Geometry: final body of the model. Coordinates: model frame, mm. A direction names the side the tool comes from. Give positions to 0.01 mm unless a question says otherwise; leave off trailing zeros. Order: outer loops, then holes, each group sorted by start corner. A loop starts at its lowest first (then second) coordinate and runs counter-clockwise, first axis right, second up. Notation, with made-up numbers: (-4, -23) -> (40, -23) arc R17 ccw to (40, 3) -> close; hole circle Ø11 at (-23, 74.25). An arc over 180 degrees is marked (long way). One line per question, with ' | ' between items.
Autodesk Inventor part; units mm, degrees
ref_plane "Work Plane2" through (0, 0, -18.4174) normal (0, 0, 1) x (1, 0, 0)
ref_plane "YZ Plane" through (0, 0, 0) normal (1, 0, 0) x (0, 1, 0)
ref_plane "XZ Plane" through (0, 0, 0) normal (0, 1, 0) x (-1, 0, 0)
sketch "Sketch1" plane through (0, 0, 0) normal (0, 1, 0) x (-1, 0, 0)
  line L0 (60.406, 25.6071) -> (-60.406, 25.6071)
  line L1 (-60.406, 25.6071) -> (-60.406, -25.6071)
  line L2 (-60.406, -25.6071) -> (60.406, -25.6071)
  line L3 (60.406, -25.6071) -> (60.406, 25.6071)
  line L4 (60.406, 25.6071) -> (-60.406, -25.6071) construction
  line L5 (-60.406, 25.6071) -> (60.406, -25.6071) construction
  line L6 (-57.406, 25.6071) -> (-57.406, -25.6071)
  line L7 (57.406, -25.6071) -> (57.406, 25.6071)
  line L8 (57.406, 23.5058) -> (55.4493, 23.5058)
  line L9 (-55.4493, 23.5058) -> (-57.406, 23.5058)
  line L10 (-57.406, -33.4947) -> (-79.0126, -33.4947)
  line L11 (79.0126, -33.4947) -> (57.406, -33.4947)
  point P0 (0, 0)
  dimension "d0" = 120.812
  dimension "d1" = 51.2141
  dimension "d8" = 3
  dimension "d9" = 3
  dimension "d10" = 114.812
extrude "Extrusion1" add sketch "Sketch1" along normal blind 3
extrude "Extrusion2" add sketch "Sketch1" along normal blind 63 contours L3 L2 L7 L0 | L6 L2 L1 L0
ref_plane "Work Plane2" through (0, 0, -18.4174) normal (0, 0, 1) x (1, 0, 0)
sketch "Sketch2" plane through (0, 0, 0) normal (0, -1, 0) x (1, 0, 0)
  circle A0 centre (-50.5968, 0.5202) radius 1.75
  circle A1 centre (-28.0003, -13.4843) radius 1.75
  circle A2 centre (50.5962, 0.5202) radius 1.75
  circle A3 centre (27.9997, -13.4843) radius 1.75
  circle A4 centre (27.9997, -13.4843) radius 1.75
  circle A5 centre (50.5962, 0.5202) radius 1.75
  circle A6 centre (-28.0003, -13.4843) radius 1.75
  circle A7 centre (-50.5968, 0.5202) radius 1.75
  point P0 (0, 0)
  dimension "d12" = 3.5
  dimension "d13" = 3.5
  dimension "d14" = 3.5
  dimension "d15" = 3.5
extrude "Extrusion3" cut sketch "Sketch2" against normal up to next
sketch "Sketch4" plane through (0, 63, 0) normal (0, 1, 0) x (1, 0, 0)
  line L0 (-60.406, -8.75) -> (-56.906, -8.75)
  line L1 (-56.906, -8.75) -> (-56.906, 8.75)
  line L2 (-56.906, 8.75) -> (-60.406, 8.75)
  line L3 (-60.406, -8.75) -> (-60.406, 8.75)
  line L4 (0, 0) -> (0, 8.75)
  line L5 (60.406, -8.75) -> (56.906, -8.75)
  line L6 (56.906, -8.75) -> (56.906, 8.75)
  line L7 (56.906, 8.75) -> (60.406, 8.75)
  line L8 (60.406, -8.75) -> (60.406, 8.75)
  point P0 (-60.406, 0)
  point P1 (60.406, 0)
  dimension "d18" = 17.5
extrude "Extrusion4" cut sketch "Sketch4" against normal blind 3
sketch "Sketch6" plane through (0, 0, 0) normal (0, -1, 0) x (1, 0, 0)
  circle A0 centre (-32.4423, 8.2996) radius 1.5
  circle A1 centre (32.4417, 8.2996) radius 1.5
  point P0 (0, 0)
extrude "Extrusion5" cut sketch "Sketch6" against normal up to next
sketch "Sketch9" plane through (60.406, 0, 25.6071) normal (1, 0, 0) x (0, 0, -1)
  circle A0 centre (3, 59.0338) radius 1
  circle A1 centre (3, 38.0338) radius 1
  circle A2 centre (48.2141, 59.0338) radius 1
  circle A3 centre (48.2141, 38.0338) radius 1
  point P0 (25.6071, 0)
extrude "Extrusion7" cut sketch "Sketch9" against normal blind 200
sketch "Sketch10" plane through (0, 0, 0) normal (0, -1, 0) x (1, 0, 0)
  circle A0 centre (-28.0003, -13.4843) radius 1.75
  circle A1 centre (27.9997, -13.4843) radius 1.75
  line L0 (53.5962, 73.5112) -> (-53.5968, 73.5112)
  line L1 (-24.5003, -13.4843) -> (24.4997, -13.4843)
  line L2 (24.4997, 73.5112) -> (-24.5003, 73.5112)
  line L3 (-24.5003, -13.4843) -> (-24.5003, -2.4798)
  line L4 (-24.5003, -13.4843) -> (-13.4958, -13.4843) construction
  line L5 (-24.5003, -2.4798) -> (24.4997, -2.4798)
  line L6 (24.4997, -13.4843) -> (24.4997, -2.4798)
  point P0 (0, 0)
  dimension "d39" = 90
extrude "Extrusion8" cut sketch "Sketch10" against normal up to next contours L3 L5 L6 L1
sketch "Sketch11" plane through (0, 0, 0) normal (0, -1, 0) x (1, 0, 0)
  circle A0 centre (-38.0003, 13.0422) radius 1.75
  circle A1 centre (-14.0003, 13.0422) radius 1.75
  line L0 (-36.0003, -4.4688) -> (-36.0003, 50.5312)
  line L1 (-16.0003, 50.5312) -> (-16.0003, -4.4688)
  line L2 (-34.6078, 15.0422) -> (34.6072, 15.0422)
  point P0 (0, 0)
  dimension "d31" = 3.5
  dimension "d32" = 3.5
  dimension "d33" = 2
  dimension "d34" = 2
  dimension "d37" = 2
  dimension "d38" = 2
extrude "Extrusion9" cut sketch "Sketch11" against normal up to next
sketch "Sketch15" plane through (-60.406, 0, -25.6071) normal (-1, 0, 0) x (0, 0, 1)
  circle A0 centre (-6.7939, 16.9) radius 9.2
  point P0 (25.6071, 0)
extrude "Extrusion11" cut sketch "Sketch15" against normal through all
sketch "Sketch16" plane through (0, 0, 0) normal (0, -1, 0) x (1, 0, 0)
  line L0 (45.6757, 24.585) -> (45.6757, 11.915)
  line L1 (51.4357, 11.915) -> (51.4357, 24.585)
  line L2 (45.6757, 11.915) -> (51.4357, 11.915)
  line L3 (51.4357, 24.585) -> (45.6757, 24.585)
  line L4 (43.5557, 27) -> (53.5557, 27)
  line L5 (53.5557, 27) -> (53.5557, 9.5)
  line L6 (53.5557, 9.5) -> (43.5557, 9.5)
  line L7 (43.5557, 9.5) -> (43.5557, 27)
  line L8 (43.5557, 27) -> (53.5557, 9.5) construction
  line L9 (53.5557, 27) -> (43.5557, 9.5) construction
  point P0 (0, 0)
  point P1 (48.5557, 18.25)
  dimension "d49" = 10
  dimension "d50" = 17.5
extrude "Extrusion12" cut sketch "Sketch16" against normal up to next contours L3 L1 L2 L0 | L4 L5 L6 L7
sketch "Sketch17" plane through (0, 3, 0) normal (0, 1, 0) x (1, 0, 0)
  circle A0 centre (-28.0003, 13.4843) radius 1.75
  circle A1 centre (27.9997, 13.4843) radius 1.75
  circle A2 centre (-28.0003, 7.4843) radius 1.75
  circle A3 centre (27.9997, 7.4843) radius 1.75
  line L0 (-24.5003, 13.4843) -> (24.4997, 13.4843)
  line L1 (-24.5003, 2.4798) -> (-24.5003, 13.4843)
  circle A4 centre (-50.5968, -0.5202) radius 1.75
  circle A5 centre (50.5962, -0.5202) radius 1.75
  line L2 (-24.5003, -2.2702) -> (24.4997, -2.2702)
  line L3 (24.4997, -2.2702) -> (24.4997, 17.7298)
  line L4 (24.4997, 17.7298) -> (-24.5003, 17.7298)
  line L5 (-24.5003, 17.7298) -> (-24.5003, -2.2702)
  point P0 (0, 0)
  dimension "d53" = 3.5
  dimension "d54" = 6
  dimension "d55" = 6
  dimension "d56" = 20
sketch "Sketch18" plane through (-60.406, 0, -25.6071) normal (-1, 0, 0) x (0, 0, 1)
  circle A0 centre (5, 31.008) radius 1
  line L0 (0, 0) -> (51.2141, 0)
  line L1 (0, 23.1035) -> (0, 63)
  circle A1 centre (5.7141, 5.5) radius 1
  line L2 (0, 0) -> (0, 10.6965)
  point P0 (25.6071, 0)
  dimension "d59" = 5
  dimension "d60" = 2
  dimension "d61" = 5.5
  dimension "d62" = 5.7141
extrude "Extrusion13" cut sketch "Sketch18" against normal through all
extrude "Extrusion14" cut sketch "Sketch17" against normal through all contours A2 | A3 | L5 L4 L3 L0 | L0 L3 L2 L5 L1
equation "\"d55\" = d54"
properties part number "Kepala Tengah 2"
1) Section A-A on z = -2.5. Return loops of the section in (x, y).
Check result:
outline: (-60.41, 0) -> (-24.5, 0) -> (-24.5, 3) -> (-57.41, 3) -> (-57.41, 60) -> (-60.41, 60) -> close; (24.5, 0) -> (60.41, 0) -> (60.41, 60) -> (57.41, 60) -> (57.41, 3) -> (24.5, 3) -> close
2) Set-up query: faces 1 (the flat face through (59, 60, 0)), 2 (the flat face through (24.5, 2, -8)), 3 (the flat face through (49, 1, 9.5)), 4 (the flat face through (57.406, 33, 0)). Return all of +Z, -Z, +X, -X, +Y, -Y with unobstructed straight access to the full face (end or side cutting, diameter ignored); none if empty.
Check result:
face 1: +X, -X, +Y | face 2: +Y, -Y | face 3: +Z, +Y, -Y | face 4: +Z, -Z, +Y
3) Section C-C on z = 5.5. Return loops of the section in (x, y).
Check result:
outline: (-60.41, 0) -> (60.41, 0) -> (60.41, 60) -> (57.41, 60) -> (57.41, 3) -> (-57.41, 3) -> (-57.41, 60) -> (-60.41, 60) -> close
4) Pull-direction query (Z, two-part tool) for faces 5 (the flat face through (60.406, 31, 0)), 6 (the flat face through (0, 2, -25.607)), 7 (the flat face through (-59, 62, -8.75)); classes: +Z half, -Z half, draft (parallel to the pull), parting line (faces both ways), or undercut.
Check result:
face 5: draft | face 6: -Z half | face 7: undercut
5) Contact query for flat-ended pins moving along their axis: pin 1 Ø2.5 at (x, z) = (-58.5, 2.5) entering from +Y; pin 2 Ø0.9 at (x, y) = (50.5, 1) entering from +Z. Output: stop coordinate, or through.
Check result:
pin 1: stops at y = 60 | pin 2: stops at z = 9.5
6) Material intervals for probe 1 along X at (y, z) = (32, -5); probe 2 along Y at (x, z) = (-14, 21); probe 3 along Z at (x, y) = (-58, 5), sorted ascending. Write a range as from..to.
Check result:
probe 1: x = -60.41..-57.41, 57.41..60.41 | probe 2: y = 0..3 | probe 3: z = -25.61..-20.76, -19.03..25.61
7) Section D-D on y = 21. Return loops of the section in (x, z), plus the area to 3 significant figures.
Check result:
outline: (-60.41, -24.17) -> (-57.41, -24.17) -> (-57.41, 25.61) -> (-60.41, 25.61) -> close; (57.41, -24.17) -> (60.41, -24.17) -> (60.41, 25.61) -> (57.41, 25.61) -> close | area: 299 mm^2
8) Section B-B on y = 55. Return loops of the section in (x, z).
Check result:
outline: (-60.41, -25.61) -> (-57.41, -25.61) -> (-57.41, 25.61) -> (-60.41, 25.61) -> close; (57.41, -25.61) -> (60.41, -25.61) -> (60.41, 25.61) -> (57.41, 25.61) -> close
